Work out the finished part from the listing and answer in its coordinate system (mm). Round coordinates to 2 decimals unless told otherwise and drop trailing zeros. Write each loop counter-clockwise with the first axis right and the second up, starting at its lowest first coordinate (ties: lowest second). Pieces come first, ordered by that corner, then holes. Notation, with made-up numbers: M 59,80 L 67,80 A9 ccw 67,94 Z; hole C -28,27.25 d6. An arc over 180 degrees is marked long. One line per item, written item: value. Start each with the question number.
Q1. Consider probe 1 along X at (y, z) = (-1, 0); probe 2 along Z at (x, y) = (-25, -1); probe 3 along X at (y, z) = (-1.4, -17.5). Determine where each line is inside the solid, lowest interval first.
Q2. The mould has two halves that part along X. Classify faces 1 (the cylindrical face through (-30, -0.99, -51.96)), 2 (the cylindrical face through (-40.92, -0.99, -23.76)), 3 (the flat face through (-28, -2, -13)): released by +X, released by -X, zero draft, split by the parting line, or undercut.
Q3. Find section B-B (x = 10). Write down the section's boundary in (y, z), and give its area (3 significant figures).
Q4. Given pin 1 Ø2.5 at (x, z) = (-25, 43.3) entering from -Y; pin 2 Ø1 at (y, z) = (-0.5, -20.5) entering from +X, each flat-ended and moving along its own axis, determine where each tip first touches the part or whether it passes through.
Q5. Find section A-A (z = 0). Write down the section's boundary in (x, y), and give its area (3 significant figures).
Q6. Find section C-C (z = 13.5). Write down the section's boundary in (x, y), and give its area (3 significant figures).
Q7. Find section D-D (y = -0.35). Write down the section's boundary in (x, z).
from build123d import *

# Parameters (mm, degrees)
SKETCH1_R           = 30
SKETCH1_R_2         = 1.5
BOSS_EXTRUDE1_DEPTH = 2


with BuildPart() as part:
    # Sketch1 → Boss-Extrude1 (new body)
    with BuildSketch(Plane(origin=(0, 0, 0), x_dir=(1, 0, 0), z_dir=(0, 1, 0))):
        with BuildLine():
            ThreePointArc((-34.962941109, -42.441151321), (-29.8558191, -52.043181929), (-19.005152341, -51.305131854))
            ThreePointArc((-19.005152341, -51.305131854), (0.154978651, -47.316486178), (19.273644656, -51.499370852))
            ThreePointArc((19.273644656, -51.499370852), (30.142808095, -51.877488756), (34.928971359, -42.111510658))
            ThreePointArc((34.928971359, -42.111510658), (41.054768373, -23.52402764), (54.236585765, -9.05821953))
            ThreePointArc((54.236585765, -9.05821953), (59.998627194, 0.165693174), (53.934123701, 9.193621197))
            ThreePointArc((53.934123701, 9.193621197), (40.899789722, 23.792458538), (34.962941109, 42.441151321))
            ThreePointArc((34.962941109, 42.441151321), (29.8558191, 52.043181929), (19.005152341, 51.305131854))
            ThreePointArc((19.005152341, 51.305131854), (-0.154978651, 47.316486178), (-19.273644656, 51.499370852))
            ThreePointArc((-19.273644656, 51.499370852), (-30.142808095, 51.877488756), (-34.928971359, 42.111510658))
            ThreePointArc((-34.928971359, 42.111510658), (-41.054768373, 23.52402764), (-54.236585765, 9.05821953))
            ThreePointArc((-54.236585765, 9.05821953), (-59.998627194, -0.165693174), (-53.934123701, -9.193621197))
            ThreePointArc((-53.934123701, -9.193621197), (-40.899789722, -23.792458538), (-34.962941109, -42.441151321))
        make_face()
        with Locations(Location((0, 0, 0), (0, 0, 90))):
            Circle(SKETCH1_R, mode=Mode.SUBTRACT)
        with Locations(Location((50, 0, 0), (0, 0, 90))):
            Circle(SKETCH1_R_2, mode=Mode.SUBTRACT)
        with Locations(Location((25, -43.301270189, 0), (0, 0, 90))):
            Circle(SKETCH1_R_2, mode=Mode.SUBTRACT)
        with Locations(Location((25, 43.301270189, 0), (0, 0, 90))):
            Circle(SKETCH1_R_2, mode=Mode.SUBTRACT)
        with Locations(Location((-25, -43.301270189, 0), (0, 0, 90))):
            Circle(SKETCH1_R_2, mode=Mode.SUBTRACT)
        with Locations(Location((-50, 0, 0), (0, 0, 90))):
            Circle(SKETCH1_R_2, mode=Mode.SUBTRACT)
        with Locations(Location((-25, 43.301270189, 0), (0, 0, 90))):
            Circle(SKETCH1_R_2, mode=Mode.SUBTRACT)
    extrude(amount=-BOSS_EXTRUDE1_DEPTH)


solid = part.part
The answers:
1. probe 1: -60 to -51.5, -48.5 to -30, 30 to 48.5, 51.5 to 60
1. probe 2: -53.3 to -44.8, -41.8 to -16.58, 16.58 to 41.8, 44.8 to 53.3
1. probe 3: -45.24 to -24.37, 24.37 to 45.2
2. face 1: undercut
2. face 2: released by -X
2. face 3: zero draft
3. outline: M -2,-48.38 L 0,-48.38 L 0,-28.28 L -2,-28.28 Z; M -2,28.28 L 0,28.28 L 0,48.41 L -2,48.41 Z
3. area: 80.4 mm2
4. pin 1: through
4. pin 2: x = 43.31
5. outline: M -60,-2 L -51.5,-2 L -51.5,0 L -60,0 Z; M -48.5,-2 L -30,-2 L -30,0 L -48.5,0 Z; M 30,-2 L 48.5,-2 L 48.5,0 L 30,0 Z; M 51.5,-2 L 60,-2 L 60,0 L 51.5,0 Z
5. area: 108 mm2
6. outline: M -48.85,-2 L -26.79,-2 L -26.79,0 L -48.85,0 Z; M 26.79,-2 L 48.91,-2 L 48.91,0 L 26.79,0 Z
6. area: 88.4 mm2
7. outline: M -54.24,-9.06 A46.87 cw -34.93,-42.11 A10 ccw -19.27,-51.5 A46.87 cw 19.01,-51.31 A10 ccw 34.96,-42.44 A46.87 cw 53.93,-9.19 A10 ccw 54.24,9.06 A46.87 cw 34.93,42.11 A10 ccw 19.27,51.5 A46.87 cw -19.01,51.31 A10 ccw -34.96,42.44 A46.87 cw -53.93,9.19 A10 ccw Z; hole C -50,0 d3; hole C 0,0 d60; hole C -25,-43.3 d3; hole C -25,43.3 d3; hole C 25,-43.3 d3; hole C 25,43.3 d3; hole C 50,0 d3
